Source: CAD feature listing. Evaluate the final solid. Frame: model axes, mm. A direction names the side the tool comes from. Coordinates: 2 decimals unless noted, no trailing zeros. Loops run counter-clockwise (first coordinate to the right, second up) from the corner with the lowest first, then second, coordinate; pieces in that order, holes last. Notation, with made-up numbers: (40, 58.25) -> (75, 58.25) arc R17 cw to (75, 68.25) -> close; hole circle Ø3 at (-31.5, -38). An arc over 180 degrees is marked (long way). Answer as a JSON object with one key per item and string values. Group by question number.
from build123d import *

# Parameters (mm, degrees)
F0_W     = 100
F0_H     = 100
F1_DEPTH = 50
F2_W     = 81.016191
F2_H     = 84.132194
F3_DEPTH = 45
F5_R     = 5.36646
F5_R_2   = 5.878275
F5_R_3   = 6.161524
F5_R_4   = 5.700697
F6_DEPTH = 25
F4_R     = 5.700697
F4_R_2   = 5.36646
F4_R_3   = 5.878275
F4_R_4   = 6.161524
F7_DEPTH = 19.5


with BuildPart() as f1:
    # F0 (on Front) → F1 (new body)
    with BuildSketch(Plane.XZ):
        Rectangle(F0_W, F0_H)
    extrude(amount=F1_DEPTH)

    # F2 (on face) → F3 (cut)
    with BuildSketch(Plane.XZ.offset(50)):
        with Locations((0.141635, 0.283275)):
            Rectangle(F2_W, F2_H)
    extrude(amount=-F3_DEPTH, mode=Mode.SUBTRACT)

    # F5 (on face) → F6 (cut)
    with BuildSketch(Plane.XZ.offset(5)):
        with Locations((-20.36646, 22.349372)):
            Circle(F5_R)
        with Locations((20.649731, 22.349372)):
            Circle(F5_R_2)
        with Locations((20.649731, -21.782822)):
            Circle(F5_R_3)
        with Locations((-20.36646, -21.782822)):
            Circle(F5_R_4)
    extrude(amount=-F6_DEPTH, mode=Mode.SUBTRACT)

    # F4 (on face) → F7 (cut)
    with BuildSketch(Plane.XZ.offset(5)):
        with Locations((-20.36646, -21.782822)):
            Circle(F4_R)
        with Locations((-20.36646, 22.349372)):
            Circle(F4_R_2)
        with Locations((20.649731, 22.349372)):
            Circle(F4_R_3)
        with Locations((20.649731, -21.782822)):
            Circle(F4_R_4)
    extrude(amount=-F7_DEPTH, mode=Mode.SUBTRACT)


solid = f1.part
1. Pin query (flat end, axial travel): pin 1 Ø1 at (x, z) = (-21.5, 17.5) entering from -Y. Return the tip coordinate at first contact, or that it passes through.
2. Reachability of faces 1 (the face through (0, -28, 42.349)), 2 (the face through (15.76, -2.54, -25.53)) from +Z, -Z, +X, -X, +Y, -Y: full face, straight path, thin tool, end or side. Return the list, or none.
3. Mould query, pull axis X, two halves, no side actions, for faces 3 (the face through (-1, -25, 50)), 4 (the face through (-50, -25, -1)), 5 (the face through (0, -28, -41.783)). Classes: pulls with the +X half, pulls with the -X half, needs draft (parallel to the pull), parting line crosses it, or undercut.
4. Section query A-A on z = -23.5. Return loops of the section in (x, y).
5. Ray query, L1, parallel to X at y = -42, z = 9.5; L2, parallel to Z at x = -29, y = -14.5; L3, parallel to Y at x = 9, z = -40. Return the intervals inside material, ascending.
6. Section query D-D on z = 12. Return loops of the section in (x, y), then the cut area to 3 significant figures.
7. Section query C-C on x = -30. Return loops of the section in (y, z), then the cut area to 3 significant figures.
8. Section query B-B on y = -42.5. Return loops of the section in (x, z), then the cut area to 3 significant figures.
Solved:
{
 "1": {"pin 1": "y = -5"},
 "2": {"face 1": "-Y", "face 2": "+Y, -Y"},
 "3": {"face 3": "needs draft", "face 4": "pulls with the -X half", "face 5": "undercut"},
 "4": {"outline": "(-50, -50) -> (-40.37, -50) -> (-40.37, -5) -> (-25.8, -5) -> (-25.8, 0) -> (-50, 0) -> close; (-14.93, -5) -> (14.73, -5) -> (14.73, 0) -> (-14.93, 0) -> close; (26.57, -5) -> (40.65, -5) -> (40.65, -50) -> (50, -50) -> (50, 0) -> (26.57, 0) -> close"},
 "5": {"L1": "-50 to -40.37, 40.65 to 50", "L2": "-50 to -41.78, 42.35 to 50", "L3": "-5 to 0"},
 "6": {"outline": "(-50, -50) -> (-40.37, -50) -> (-40.37, -5) -> (40.65, -5) -> (40.65, -50) -> (50, -50) -> (50, 0) -> (-50, 0) -> close", "area": "1,350 mm^2"},
 "7": {"outline": "(-50, -50) -> (0, -50) -> (0, 50) -> (-50, 50) -> (-50, 42.35) -> (-5, 42.35) -> (-5, -41.78) -> (-50, -41.78) -> close", "area": "1,210 mm^2"},
 "8": {"outline": "(-50, -50) -> (50, -50) -> (50, 50) -> (-50, 50) -> close; hole (-40.37, -41.78) -> (40.65, -41.78) -> (40.65, 42.35) -> (-40.37, 42.35) -> close", "area": "3,180 mm^2"}
}
